```python
from build123d import *

# Parameters (mm, degrees)
SKETCH1_R           = 75
BOSS_EXTRUDE1_DEPTH = 50
SKETCH2_R           = 50
BOSS_EXTRUDE2_DEPTH = 20
SKETCH3_R           = 15
BOSS_EXTRUDE3_DEPTH = 15
FILLET1_R           = 5


with BuildPart() as part:
    # Sketch1 → Boss-Extrude1 (new body)
    with BuildSketch(Plane.XY):
        Circle(SKETCH1_R)
    extrude(amount=BOSS_EXTRUDE1_DEPTH)

    # Sketch2 → Boss-Extrude2 (add)
    with BuildSketch(Plane.XY.offset(50)):
        Circle(SKETCH2_R)
    extrude(amount=BOSS_EXTRUDE2_DEPTH)

    # Sketch3 → Boss-Extrude3 (add)
    with BuildSketch(Plane.XY.offset(70)):
        Circle(SKETCH3_R)
    extrude(amount=BOSS_EXTRUDE3_DEPTH)

    # Fillet1
    fillet1_edges = [part.edges().sort_by_distance(p)[0] for p in [
        (-75, 0, 50),
        (-50, 0, 50),
        (-50, 0, 70),
    ]]
    fillet(fillet1_edges, radius=FILLET1_R)


solid = part.part
```
Model file for the job. Use its own axes, mm. A direction names the side the tool comes from. Coordinates: 2 decimals unless noted, no trailing zeros. Order: outer loops, then holes, each group sorted by start corner. A loop starts at its lowest first (then second) coordinate and runs counter-clockwise, first axis right, second up. Notation, with made-up numbers: (30.25, 66) -> (41.25, 66) arc R27 ccw to (41.25, 88) -> close; hole circle Ø10 at (52, 33). An arc over 180 degrees is marked (long way). Return JSON: item names as keys, results as strings.
Item 1: Slice it at A-A (y = 0). Write the cut outline in (x, z).
Model answer:
{"outline": "(-75, 0) -> (75, 0) -> (75, 45) arc R5 ccw to (70, 50) -> (55, 50) arc R5 cw to (50, 55) -> (50, 65) arc R5 ccw to (45, 70) -> (15, 70) -> (15, 85) -> (-15, 85) -> (-15, 70) -> (-45, 70) arc R5 ccw to (-50, 65) -> (-50, 55) arc R5 cw to (-55, 50) -> (-70, 50) arc R5 ccw to (-75, 45) -> close"}
Item 2: 3-axis set-ups, long thin cutter, end or side, ignore diameter. For faces 1 (the face through (47.69, 15.02, 59.93)), 2 (the face through (-1, 1, 0)): which of +Z, -Z, +X, -X, +Y, -Y reach the whole face in a straight line?
Model answer:
{"face 1": "+Z", "face 2": "-Z, +X, -X, +Y, -Y"}
Item 3: Slice it at C-C (z = 39). Write the cut outline in (x, y).
Model answer:
{"outline": "circle Ø150 at (0, 0)"}
Item 4: Wall check: line 1 along Z through (x, y) = (10, -36); line 2 along Z through (x, y) = (54, 30); line 3 along X through (y, z) = (51, 24). Give the ranges that are in metal, low to high. Write a range as from..to.
Model answer:
{"line 1": "z = 0..70", "line 2": "z = 0..50", "line 3": "x = -54.99..54.99"}
Item 5: Pin check, flat tips, straight feed: P1, Ø2, axis at x = -34, y = 3, coming from the -Z side; P2, Ø1.5, axis at x = -27.5, z = 10, coming from the +Y side; P3, Ø8, axis at x = -1, y = 50, coming from the +Z side; P4, Ø8, axis at y = -16, z = 28.5, coming from the +X side. Stop position of each tip, or through.
Model answer:
{"P1": "stops at z = 0", "P2": "stops at y = 70.07", "P3": "stops at z = 69.9", "P4": "stops at x = 74.03"}
